Source: CAD feature listing. Evaluate the final solid. Frame: model axes, mm. Face numbers are marked on the shaded views. Give positions to 0.01 mm unless a question says otherwise; leave off trailing zeros. Order: outer loops, then holes, each group sorted by start corner. A loop starts at its lowest first (then second) coordinate and runs counter-clockwise, first axis right, second up. Notation, with made-up numbers: (72.5, 12.5) - (115.5, 12.5) arc R16 cw to (115.5, 28.5) - close; hole circle Ø6 at (39, -38). An arc over 180 degrees is marked (long way). Use CSV: the item, a comma, the result in double quotes.
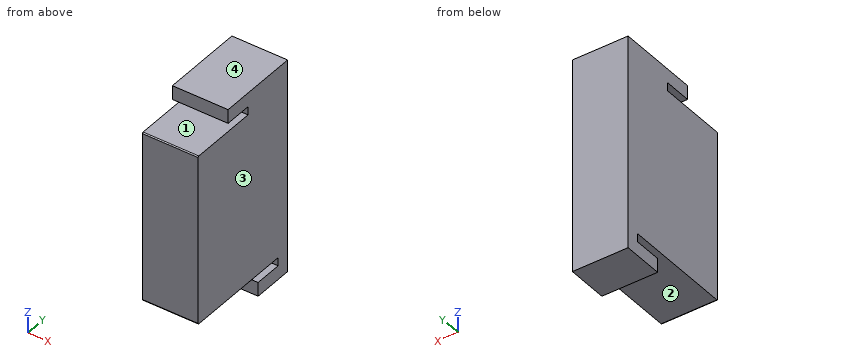
Autodesk Inventor part; units mm, degrees
ref_plane "YZ Plane" through (0, 0, 0) normal (1, 0, 0) x (0, 1, 0)
ref_plane "XZ Plane" through (0, 0, 0) normal (0, 1, 0) x (-1, 0, 0)
ref_plane "XY Plane" through (0, 0, 0) normal (0, 0, 1) x (1, 0, 0)
sketch "Sketch1" plane through (0, 0, 0) normal (1, 0, 0) x (0, 1, 0)
  line L0 (92.1534, 119.6677) -> (119.9664, 119.6677) construction
  arc A0 (92.1534, 119.6677) -> (91.3914, 118.9057) centre (92.1534, 118.9057) ccw construction
  line L1 (91.3914, 118.9057) -> (91.3914, 42.1977) construction
  arc A1 (91.3914, 42.1977) -> (92.1534, 41.4357) centre (92.1534, 42.1977) ccw construction
  line L2 (139.0164, 41.4357) -> (92.1534, 41.4357) construction
  line L3 (148.5414, 119.3677) -> (92.1534, 119.3677)
  arc A2 (92.1534, 119.3677) -> (91.6914, 118.9057) centre (92.1534, 118.9057) ccw
  line L4 (91.6914, 118.9057) -> (91.6914, 42.1977)
  arc A3 (91.6914, 42.1977) -> (92.1534, 41.7357) centre (92.1534, 42.1977) ccw
  line L5 (92.1534, 41.7357) -> (148.5414, 41.7357)
  line L6 (148.5414, 119.3677) -> (148.5414, 41.7357)
  line L7 (142.1914, 41.4357) -> (142.1914, 38.2607) construction
  line L8 (123.1414, 122.8427) -> (123.1414, 119.6677) construction
  line L9 (119.9664, 122.8427) -> (123.1414, 122.8427) construction
  line L10 (142.1914, 38.2607) -> (139.0164, 38.2607) construction
  line L11 (123.4414, 119.3677) -> (148.5414, 119.3677)
  line L12 (148.5414, 119.3677) -> (148.5414, 123.1427)
  line L13 (148.5414, 123.1427) -> (123.4414, 123.1427)
  line L14 (123.4414, 123.1427) -> (123.4414, 119.3677)
  line L15 (148.5414, 123.1427) -> (110.7414, 123.1427)
  line L16 (110.7414, 123.1427) -> (110.7414, 129.4927)
  line L17 (110.7414, 129.4927) -> (148.5414, 129.4927)
  line L18 (148.5414, 129.4927) -> (148.5414, 123.1427)
  line L19 (142.4914, 41.7357) -> (148.5414, 41.7357)
  line L20 (148.5414, 41.7357) -> (148.5414, 37.9607)
  line L21 (148.5414, 37.9607) -> (142.4914, 37.9607)
  line L22 (142.4914, 37.9607) -> (142.4914, 41.7357)
  line L23 (148.5414, 37.9607) -> (129.7914, 37.9607)
  line L24 (129.7914, 37.9607) -> (129.7914, 31.6107)
  line L25 (129.7914, 31.6107) -> (148.5414, 31.6107)
  line L26 (148.5414, 31.6107) -> (148.5414, 37.9607)
  point P0 (0, 0)
  dimension "d0" = 0.3
  dimension "d1" = 6.35
  dimension "d2" = 0.3
  dimension "d3" = 0.3
  dimension "d4" = 0.3
  dimension "d5" = 0.3
  dimension "d6" = 6.35
  dimension "d7" = 6.35
  dimension "d8" = 12.7
  dimension "d9" = 12.7
extrude "Extrusion1" add sketch "Sketch1" along normal blind 25.4
equation "\"d2\" = d0"
equation "\"d3\" = d0"
equation "\"d4\" = d0"
equation "\"d5\" = d0"
properties part number "BumperFrameStandoff"
Item 1: Section C-C on y = 106.5. Return the cut outline in (x, z), then the cut area to 3 significant figures.
Filled in:
outline,"(0, 41.74) - (25.4, 41.74) - (25.4, 119.37) - (0, 119.37) - close"
area,"1,970 mm2"
Item 2: First-contact query: pin 1 (1.5 mm diameter, centred on x = 22.5, y = 122, fed in from -Z); pin 2 (3 mm diameter, centred on x = 18.5, z = 121.5, fed in from -Y); pin 3 (3 mm diameter, centred on x = 12.5, z = 34.5, fed in from -Y). Flat tips, straight axial feed; report the tip coordinate or a pass-through.
Filled in:
pin 1,"stops at z = 41.74"
pin 2,"stops at y = 123.44"
pin 3,"stops at y = 129.79"
Item 3: Section A-A on y = 119. Return the cut outline in (x, z), then the cut area to 3 significant figures.
Filled in:
outline,"(0, 41.74) - (25.4, 41.74) - (25.4, 119.37) - (0, 119.37) - close; (0, 123.14) - (25.4, 123.14) - (25.4, 129.49) - (0, 129.49) - close"
area,"2,130 mm2"
Item 4: Material intervals for line 1 (Z direction, x = 19, y = 134); line 2 (Z direction, x = 22.5, y = 120); line 3 (Z direction, x = 6, y = 102.5), sorted ascending. Write a range as from..to.
Filled in:
line 1,"z = 31.61..37.96, 41.74..129.49"
line 2,"z = 41.74..119.37, 123.14..129.49"
line 3,"z = 41.74..119.37"
Item 5: Section B-B on x = 20.5. Return the cut outline in (y, z).
Filled in:
outline,"(91.69, 42.2) arc R0.46 ccw to (92.15, 41.74) - (142.49, 41.74) - (142.49, 37.96) - (129.79, 37.96) - (129.79, 31.61) - (148.54, 31.61) - (148.54, 129.49) - (110.74, 129.49) - (110.74, 123.14) - (123.44, 123.14) - (123.44, 119.37) - (92.15, 119.37) arc R0.46 ccw to (91.69, 118.91) - close"
Item 6: Mould query, pull axis Z, two halves, no side actions, for the marked faces 1, 2, 3 and 4. Classes: released by +Z, released by -Z, zero draft, split by the parting line, or undercut.
Filled in:
face 1,"undercut"
face 2,"undercut"
face 3,"zero draft"
face 4,"released by +Z"
